from build123d import *

# Parameters (mm, degrees)
SKETCH2_R           = 3.175
SKETCH2_R_2         = 2.413
BOSS_EXTRUDE2_DEPTH = 3.175


with BuildPart() as part:
    # Sketch2 → Boss-Extrude2 (new body)
    with BuildSketch(Plane(origin=(0, 0, 0), x_dir=(1, 0, 0), z_dir=(0, 1, 0))):
        with BuildLine():
            ThreePointArc((-57.15, -7.62), (-56.616270879, -7.601284972), (-56.085163479, -7.545231818))
            Line((-56.085163479, -7.545231818), (-44.001957312, -5.839964235))
            ThreePointArc((-44.001957312, -5.839964235), (-42.617088962, -5.579674967), (-41.261668847, -5.194386554))
            ThreePointArc((-41.261668847, -5.194386554), (-4.750522579, 3.228025881), (32.696434157, 4.541899627))
            ThreePointArc((32.696434157, 4.541899627), (39.058772614, 3.180733721), (44.734603501, 0))
            Line((44.734603501, 0), (52.473194068, -6.015969271))
            ThreePointArc((52.473194068, -6.015969271), (54.677884089, -7.207845928), (57.15, -7.62))
            ThreePointArc((57.15, -7.62), (64.357845928, -2.472115911), (61.826805932, 6.015969271))
            Line((61.826805932, 6.015969271), (54.088215365, 12.031938542))
            ThreePointArc((54.088215365, 12.031938542), (40.899560171, 18.575357931), (26.203429573, 19.458935064))
            Line((26.203429573, 19.458935064), (-58.214836521, 7.545231818))
            ThreePointArc((-58.214836521, 7.545231818), (-64.751284972, -0.533729121), (-57.15, -7.62))
        make_face()
        with Locations(Location((-57.15, 0, 0), (0, 0, 270))):
            Circle(SKETCH2_R, mode=Mode.SUBTRACT)
        with Locations(Location((57.15, 0, 0), (0, 0, 270))):
            Circle(SKETCH2_R_2, mode=Mode.SUBTRACT)
    extrude(amount=BOSS_EXTRUDE2_DEPTH)


solid = part.part
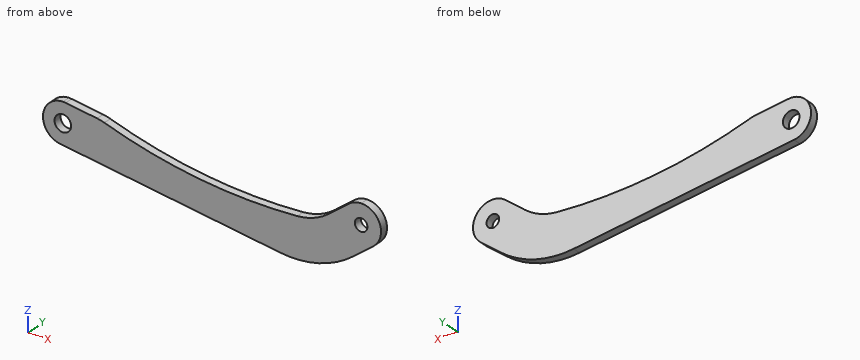
Here's how the part is built. I have some questions about the finished solid (model axes, mm). Round coordinates to 2 decimals unless told otherwise and drop trailing zeros. Write each loop counter-clockwise with the first axis right and the second up, starting at its lowest first coordinate (ties: lowest second). Pieces come first, ordered by that corner, then holes.
1. Suppose I cut it at B-B (x = 14.5). List the corners of the cut face in (y, z) for me (1 decimal).
2. Will these pins go through, and if not, where does the flat tip stop? pin 1 Ø5.5 at (x, z) = (-57.15, 0) entering from +Y; pin 2 Ø1 at (x, y) = (-51, 2) entering from +Z; pin 3 Ø1.5 at (x, z) = (-48, 1.5) entering from -Y; pin 4 Ø1.5 at (x, y) = (41.5, 1.5) entering from -Z.
3. Suppose I cut it at C-C (z = -10.5). List the corners of the cut face in (x, y) for me (3 decimals).
4. I need wall thicknesses on L1, parallel to Z at x = -59, y = 3.05; L2, parallel to Z at x = 59, y = 0.3; L3, parallel to Z at x = -40.5, y = 1.9. Which ranges of each line are inside material? Lowest first, please.
5. Suppose I cut it at A-A (y = 1.9). List the corners of the cut face in (x, z) for me (3 decimals).
Answer sheet:
1. outline: (0, -17.8) - (3.2, -17.8) - (3.2, -4.8) - (0, -4.8) - close
2. pin 1: passes through
2. pin 2: stops at z = 6.9
2. pin 3: stops at y = 0
2. pin 4: stops at z = -18.61
3. outline: (-37.278, 0) - (56.059, 0) - (56.059, 3.175) - (-37.278, 3.175) - close
4. L1: z = -7.39 to -2.58, 2.58 to 7.39
4. L2: z = -8.21 to -1.55, 1.55 to 7.39
4. L3: z = -10.05 to 4.94
5. outline: (-58.215, -7.545) - (26.203, -19.459) arc R37.007 ccw to (54.088, -12.032) - (61.827, -6.016) arc R7.62 ccw to (52.473, 6.016) - (44.735, 0) arc R21.767 cw to (32.696, -4.542) arc R195.82 cw to (-41.262, 5.194) arc R15.462 ccw to (-44.002, 5.84) - (-56.085, 7.545) arc R7.62 ccw to start; hole circle Ø6.35 at (-57.15, 0); hole circle Ø4.826 at (57.15, 0)
